```python
from build123d import *

# Parameters (mm, degrees)
SKETCH_1_R      = 1.8
EXTRUDE_1_REACH = 30.75
SKETCH_2_R      = 1.8
SKETCH_3_R      = 1.5
EXTRUDE_2_DEPTH = 16


with BuildPart() as part:
    # 草图1 → 旋转1 (revolve)
    with BuildSketch(Plane.XY):
        with Locations((-3.95, 0)):
            Circle(SKETCH_1_R)
    revolve(axis=Axis((0, 9.659818304, 0), (0, -1, 0)))

    # 草图2 → 凸台-拉伸1 (add, up to next)
    with BuildSketch(Plane.XY.offset(23), mode=Mode.PRIVATE) as extrude_1_sk1:
        Circle(SKETCH_2_R)
    extrude_1_tool1 = extrude(extrude_1_sk1.sketch, amount=-EXTRUDE_1_REACH, mode=Mode.PRIVATE) - part.part
    add(extrude_1_tool1.solids().sort_by_distance((0, 0, 23))[0])

    # 草图3 → 凸台-拉伸2 (add)
    with BuildSketch(Plane.XY.offset(23)):
        Circle(SKETCH_3_R)
    extrude(amount=EXTRUDE_2_DEPTH)


solid = part.part
```
The model under review builds one solid part; all positions refer to its coordinate system, in mm. A direction names the side the tool comes from. Round coordinates to 2 decimals unless told otherwise and drop trailing zeros. Write each loop counter-clockwise with the first axis right and the second up, starting at its lowest first coordinate (ties: lowest second). Pieces come first, ordered by that corner, then holes.
(1) We need section A-A on x = 0. Give the boundary of the cut face in (y, z), and give its area (3 significant figures).
(2) We need section D-D on z = 32. Give the boundary of the cut face in (x, y), and give its area (3 significant figures).
(3) Wall thickness on L1, parallel to Z at x = 0, y = 1.55; L2, parallel to Z at x = 1.5, y = 0.5; L3, parallel to X at y = 0.15, z = -1.5: over which ranges is each line inside the solid? List them lowest first.
(4) Machinability: for faces 1 (the flat face through (0, 0, 39)), 2 (the cylindrical face through (-1.5, 0.07, 30.89)), which of the approach directions +Z, -Z, +X, -X, +Y, -Y give a long, thin tool a straight path to every point of the face, cutting with its end or side? Answer none if there is none.
(5) Insertion check: pin 1 (6 mm diameter, centred on x = 4, z = 3, fed in from +Y); pin 2 (3 mm diameter, centred on x = -2.5, z = 14, fed in from +Y); pin 3 (3 mm diameter, centred on x = -3, z = 11, fed in from -Y) (3 decimals). Each pin has a flat end and moves straight along its axis. Give the tip position at first contact, or say it passes through.
(6) We need section B-B on y = 0. Give the boundary of the cut face in (x, z), and give its area (3 significant figures).
(7) We need section C-C on z = 10. Give the boundary of the cut face in (x, y), and give its area (3 significant figures).
Findings below:
1. outline: circle Ø3.6 at (0, -3.95); (-1.8, 3.95) arc R1.8 ccw to (1.8, 3.95) - (1.8, 23) - (1.5, 23) - (1.5, 39) - (-1.5, 39) - (-1.5, 23) - (-1.8, 23) - close
1. area: 132 mm2
2. outline: circle Ø3 at (0, 0)
2. area: 7.07 mm2
3. L1: z = -4.87 to -3.03, 3.03 to 23
3. L2: z = -5.48 to -1.64, 1.64 to 23
3. L3: x = -5.54 to -1.55, 1.55 to 5.54
4. face 1: +Z, +X, -X, +Y, -Y
4. face 2: +Z
5. pin 1: stops at y = 1.8
5. pin 2: stops at y = 1.5
5. pin 3: stops at y = -0.995
6. outline: (-1.8, 5.46) arc R5.75 ccw (long way) to (1.8, 5.46) - (1.8, 23) - (1.5, 23) - (1.5, 39) - (-1.5, 39) - (-1.5, 23) - (-1.8, 23) - close; hole circle Ø4.3 at (0, 0)
6. area: 200 mm2
7. outline: circle Ø3.6 at (0, 0)
7. area: 10.2 mm2
